```python
from build123d import *

# Parameters (mm, degrees)
F1_DEPTH = 6.35
F2_W     = 5.08
F2_H     = 63.5
F3_DEPTH = 127
F4_R     = 3.175
F5_DEPTH = 50.8


with BuildPart() as f1:
    # F0 (on Top) → F1 (new body)
    with BuildSketch(Plane.XY):
        with BuildLine():
            ThreePointArc((38.1, 0), (19.05, -19.05), (0, 0))
            Line((0, 0), (0, -63.5))
            ThreePointArc((0, -63.5), (19.05, -44.45), (38.1, -63.5))
            Line((38.1, -63.5), (38.1, 0))
        make_face()
        with BuildLine():
            ThreePointArc((38.1, 0), (19.05, 19.05), (0, 0))
            ThreePointArc((0, 0), (19.05, -19.05), (38.1, 0))
        make_face()
        with BuildLine():
            ThreePointArc((38.1, -63.5), (19.05, -44.45), (0, -63.5))
            ThreePointArc((0, -63.5), (19.05, -82.55), (38.1, -63.5))
        make_face()
    extrude(amount=F1_DEPTH)

    # F2 (on face) → F3 (join)
    with BuildSketch(Plane.XY.offset(6.35)):
        with Locations((2.54, -31.75)):
            Rectangle(F2_W, F2_H)
        with Locations((35.56, -31.75)):
            Rectangle(F2_W, F2_H)
    extrude(amount=F3_DEPTH)

    # F4 (on face) → F5 (cut)
    with BuildSketch(Plane.YZ.offset(38.1)):
        with Locations((-31.75, 120.65)):
            Circle(F4_R)
        with Locations((-31.75, 82.55)):
            Circle(F4_R)
        with Locations((-38.1, 38.1)):
            Circle(F4_R)
    extrude(amount=-F5_DEPTH, mode=Mode.SUBTRACT)


solid = f1.part
```
CAD build for the part. Positions are in the model's coordinates, mm. A direction names the side the tool comes from. Coordinates: 2 decimals unless noted, no trailing zeros. Loops run counter-clockwise (first coordinate to the right, second up) from the corner with the lowest first, then second, coordinate; pieces in that order, holes last. Notation, with made-up numbers: (-26.5, -36) - (-14.5, -36) arc R19 cw to (-14.5, -4) - close; hole circle Ø11 at (79, 43). An arc over 180 degrees is marked (long way). Use CSV: the item, a comma, the result in double quotes. Start each with the question number.
Q1. Cut at A-A, the plane z = 46.5. List the corners of the cut face in (x, y), then the cut area to 3 significant figures.
Q2. Probe probe 1 along X at (y, z) = (-58, 86); probe 2 along Z at (x, y) = (6, 12); probe 3 along Y at (x, z) = (35.5, 23.5). List the from-to ranges inside material, lowest first. Write a range as from..to.
Q3. 3-axis set-ups, long thin cutter, end or side, ignore diameter. For faces 5 (the flat face through (33.02, -32, 69)), 6 (the flat face through (3, 0, 69)), 7 (the flat face through (36, -63.5, 69)): which of +Z, -Z, +X, -X, +Y, -Y reach the whole face in a straight line?
Q4. Cut at D-D, the plane y = -55. List the corners of the cut face in (x, z), then the cut area to 3 significant figures.
Q5. Cut at C-C, the plane x = 35.5. List the corners of the cut face in (y, z) (3 decimals), then the cut area to 3 significant figures.
Q6. Drop flat-ended pins along their axis: P1, Ø1.5, axis at x = 36.5, z = 79.5, coming from the +Y side; P2, Ø1, axis at x = 6, y = -50.5, coming from the +Z side; P3, Ø2.5, axis at x = 36, z = 50, coming from the -Y side. Give the stop position or say it passes through.
Q7. Two-plate mould, pull along Y, no slides. Class faces 1 (the flat face through (36, -31, 133.35)), 2 (the flat face through (3, -63.5, 69)), 3 (the cylindrical face through (2.58, -32.44, 117.55)), 4 (the cylindrical face through (35.6, -32.44, 117.55)): +Y half, -Y half, draft (parallel to the pull), parting line (faces both ways), or undercut.
Q8. Cut at B-B, the plane z = 120.65. List the corners of the cut face in (x, y) (3 decimals).
Here are the results:
1,outline,"(0, -63.5) - (5.08, -63.5) - (5.08, 0) - (0, 0) - close; (33.02, -63.5) - (38.1, -63.5) - (38.1, 0) - (33.02, 0) - close"
1,area,"645 mm2"
2,probe 1,"0..5.08, 33.02..38.1"
2,probe 2,"0..6.35"
2,probe 3,"-63.5..0"
3,face 5,"+Z, +Y, -Y"
3,face 6,"+Z, +X, -X, +Y"
3,face 7,"+Z, +X, -X, -Y"
4,outline,"(0, 0) - (38.1, 0) - (38.1, 133.35) - (33.02, 133.35) - (33.02, 6.35) - (5.08, 6.35) - (5.08, 133.35) - (0, 133.35) - close"
4,area,"1,530 mm2"
5,outline,"(-73.107, 0) - (9.607, 0) - (9.607, 6.35) - (0, 6.35) - (0, 133.35) - (-63.5, 133.35) - (-63.5, 6.35) - (-73.107, 6.35) - close; hole circle Ø6.35 at (-38.1, 38.1); hole circle Ø6.35 at (-31.75, 82.55); hole circle Ø6.35 at (-31.75, 120.65)"
5,area,"8,490 mm2"
6,P1,"y = 0"
6,P2,"z = 6.35"
6,P3,"y = -63.5"
7,face 1,"draft"
7,face 2,"-Y half"
7,face 3,"undercut"
7,face 4,"undercut"
8,outline,"(0, -63.5) - (5.08, -63.5) - (5.08, -34.925) - (0, -34.925) - close; (0, -28.575) - (5.08, -28.575) - (5.08, 0) - (0, 0) - close; (33.02, -63.5) - (38.1, -63.5) - (38.1, -34.925) - (33.02, -34.925) - close; (33.02, -28.575) - (38.1, -28.575) - (38.1, 0) - (33.02, 0) - close"
